Here's how the part is built. I have some questions about the finished solid (model axes, mm). A direction names the side the tool comes from. Give positions to 0.01 mm unless a question says otherwise; leave off trailing zeros. Write each loop counter-clockwise with the first axis right and the second up, starting at its lowest first coordinate (ties: lowest second). Pieces come first, ordered by that corner, then holes. Notation, with made-up numbers: (6.5, 5) - (17.5, 5) arc R7 ccw to (17.5, 12) - close; hole circle Ø4 at (-29, 48). An arc over 180 degrees is marked (long way). Write each question's results on one line, items separated by ' | '. Start each with the question number.
Item 1: Suppose I cut it at A-A on y = -11.75. List the corners of the cut face in (x, z) for me, then the cut area to 3 significant figures.
Item 2: Suppose I cut it at B-B on x = 0. Count the separate pieces of the cut face and the enclosed holes in it, then the cut area to 3 significant figures.
Item 3: We'd pull the mould along X, two halves only. Please class faces 5 (the flat face through (0, 3, 34)), 6 (the cylindrical face through (9, 0, 89)), 7 (the flat face through (-4, 0, 88)): +X half, -X half, draft (parallel to the pull), parting line (faces both ways), or undercut.
Item 4: Suppose I cut it at D-D on y = 10.25. List the corners of the cut face in (x, z) for me, then the cut area to 3 significant figures.
Item 5: Which directions (+Z, -Z, +X, -X, +Y, -Y) give clear straight access to the entire face, cutting with the end or side of a thin tool? Please do faces 1 (the flat face through (0, -4, 88)), 2 (the cylindrical face through (-9, 0, 86)), 3 (the cylindrical face through (-1.5, 6.896, 52.117)), 4 (the flat face through (0, -1, 75)).
Item 6: Will these pins go through, and if not, where does the flat tip stop? P1, Ø10.5, axis at x = 0, z = 55, coming from the -Y side; P2, Ø2.5, axis at x = 0, z = 87.5, coming from the +Y side; P3, Ø0.9, axis at y = 0, z = 88, coming from the +X side; P4, Ø3, axis at x = -6.5, y = -7, coming from the +Z side.
Item 7: Please list where these lines run through material, in increasing order: line 1 along Z through (x, y) = (0, 6.25); line 2 along Z through (x, y) = (0, -6.8); line 3 along Z through (x, y) = (-12.5, -4).
Item 8: Suppose I cut it at C-C on z = 34.5. List the corners of the cut face in (x, y) for me.
Autodesk Inventor part; units mm, degrees
ref_plane "作業平面1" through (14, 0, 0) normal (1, 0, 0) x (0, 1, 0)
ref_plane "作業平面2" through (-14, 0, 0) normal (1, 0, 0) x (0, 1, 0)
ref_plane "作業平面3" through (0, 7.5, 0) normal (0, 1, 0) x (-1, 0, 0)
sketch "スケッチ1" plane through (0, 0, 0) normal (0, 0, 1) x (1, 0, 0)
  circle A0 centre (0, 0) radius 7.5
  dimension "d0" = 15
extrude "押し出し1" add sketch "スケッチ1" along normal blind 82.5
ref_plane "作業平面1" through (14, 0, 0) normal (1, 0, 0) x (0, 1, 0)
ref_plane "作業平面2" through (-14, 0, 0) normal (1, 0, 0) x (0, 1, 0)
ref_plane "作業平面3" through (0, 7.5, 0) normal (0, 1, 0) x (-1, 0, 0)
ref_plane "作業平面4" through (0, -7.5, 0) normal (0, 1, 0) x (-1, 0, 0)
sketch "スケッチ7" plane through (0, 7.5, 0) normal (0, 1, 0) x (-1, 0, 0)
  circle A0 centre (0, 55) radius 1.7
  line L0 (7.5, 82.5) -> (-7.5, 82.5)
  point P0 (0, 0)
  dimension "d35" = 3.4
  dimension "d87" = 27.5
extrude "押し出し7" cut sketch "スケッチ7" against normal through all
sketch "スケッチ8" plane through (0, 7.5, 0) normal (0, 1, 0) x (-1, 0, 0)
  circle A0 centre (0, 55) radius 3.25
  line L0 (7.5, 82.5) -> (-7.5, 82.5)
  point P0 (0, 0)
  dimension "d39" = 6.5
  dimension "d85" = 27.5
sketch "スケッチ9" plane through (0, -7.5, 0) normal (0, 1, 0) x (-1, 0, 0)
  circle A0 centre (0, 55) radius 3.25
  line L0 (7.5, 82.5) -> (-7.5, 82.5)
  point P0 (0, 0)
  dimension "d41" = 6.5
  dimension "d86" = 27.5
extrude "押し出し8" cut sketch "スケッチ8" against normal blind 1
extrude "押し出し9" cut sketch "スケッチ9" along normal blind 1
sketch "スケッチ10" plane through (0, 0, 82.5) normal (0, 0, 1) x (1, 0, 0)
  circle A0 centre (0, 0) radius 14
  dimension "d47" = 28
extrude "押し出し10" add sketch "スケッチ10" along normal blind 10
ref_plane "作業平面5" through (0, 14, 0) normal (0, 1, 0) x (-1, 0, 0)
ref_plane "作業平面6" through (0, -14, 0) normal (0, 1, 0) x (-1, 0, 0)
sketch "スケッチ11" plane through (0, 14, 0) normal (0, 1, 0) x (-1, 0, 0)
  circle A0 centre (0, 87.5) radius 1.5
  line L0 (14, 92.5) -> (-14, 92.5)
  point P0 (0, 0)
  dimension "d52" = 3
  dimension "d53" = 5
sketch "スケッチ12" plane through (0, -14, 0) normal (0, 1, 0) x (-1, 0, 0)
  circle A0 centre (0, 87.5) radius 1.5
  line L0 (14, 92.5) -> (-14, 92.5)
  point P0 (0, 0)
  dimension "d54" = 3
  dimension "d55" = 5
sketch "スケッチ13" plane through (-14, 0, 0) normal (1, 0, 0) x (0, 1, 0)
  circle A0 centre (0, 87.5) radius 1.5
  line L0 (14, 92.5) -> (-14, 92.5)
  point P0 (0, 0)
  dimension "d56" = 3
  dimension "d57" = 5
sketch "スケッチ14" plane through (14, 0, 0) normal (1, 0, 0) x (0, 1, 0)
  circle A0 centre (0, 87.5) radius 1.5
  line L0 (14, 92.5) -> (-14, 92.5)
  point P0 (0, 0)
  dimension "d58" = 3
  dimension "d59" = 5
extrude "押し出し11" cut sketch "スケッチ11" against normal blind 10
extrude "押し出し12" cut sketch "スケッチ12" along normal blind 10
extrude "押し出し13" cut sketch "スケッチ14" against normal blind 10
extrude "押し出し14" cut sketch "スケッチ13" along normal blind 10
thread "ねじ5"
thread "ねじ6"
thread "ねじ7"
thread "ねじ8"
sketch "スケッチ15" plane through (0, 0, 92.5) normal (0, 0, 1) x (1, 0, 0)
  circle A0 centre (7.5, 7.5) radius 1.7
  circle A1 centre (-7.5, 7.5) radius 1.7
  circle A2 centre (-7.5, -7.5) radius 1.7
  circle A3 centre (7.5, -7.5) radius 1.7
  point P0 (0, 0)
  dimension "d76" = 3.4
  dimension "d77" = 7.5
  dimension "d78" = 7.5
  dimension "d81" = 360
extrude "押し出し15" cut sketch "スケッチ15" against normal through all
sketch "スケッチ16" plane through (0, 0, 0) normal (0, 0, -1) x (-1, 0, 0)
  circle A0 centre (0, 0) radius 14
  dimension "d88" = 28
extrude "押し出し16" add sketch "スケッチ16" along normal blind 5
sketch "スケッチ17" plane through (0, 0, -5) normal (0, 0, -1) x (-1, 0, 0)
  arc A0 (-2.9394, 3) -> (2.9394, 3) centre (0, 0) ccw
  line L0 (-2.9394, 3) -> (2.9394, 3)
  dimension "d91" = 4.2
  dimension "d92" = 3
extrude "押し出し17" cut sketch "スケッチ17" against normal blind 80
properties part number "rotary_transfer_shaft_5_2" material "ステンレス鋼"
Checked values:
1) outline: (-7.61, -5) - (7.61, -5) - (7.61, 0) - (-7.61, 0) - close; (-7.61, 82.5) - (7.61, 82.5) - (7.61, 92.5) - (-7.61, 92.5) - close; hole circle Ø3 at (0, 87.5) | area: 221 mm^2
2) separate pieces: 3 | enclosed holes: 0 | area: 989 mm^2
3) face 5: undercut | face 6: draft | face 7: -X half
4) outline: (-9.54, -5) - (9.54, -5) - (9.54, 0) - (-9.54, 0) - close; (-9.54, 82.5) - (9.54, 82.5) - (9.54, 92.5) - (-9.54, 92.5) - close; hole circle Ø3 at (0, 87.5) | area: 279 mm^2
5) face 1: -Y | face 2: -X | face 3: +Y | face 4: -Z
6) P1: stops at y = -7.5 | P2: stops at y = 4 | P3: stops at x = 4 | P4: stops at z = 92.5
7) line 1: z = -5 to 53.3, 56.7 to 86, 89 to 92.5 | line 2: z = -5 to 51.75, 58.25 to 86, 89 to 92.5 | line 3: z = -5 to 0, 82.5 to 92.5
8) outline: circle Ø15 at (0, 0); hole (-2.94, 3) arc R4.2 ccw (long way) to (2.94, 3) - close
